from build123d import *

# Parameters (mm, degrees)
SKETCH1_R           = 4
BOSS_EXTRUDE1_DEPTH = 50
SKETCH2_R           = 1.5
CUT_EXTRUDE1_DEPTH  = 5
FILLET1_R           = 2
SKETCH3_R           = 1.5
CUT_EXTRUDE2_DEPTH  = 4


with BuildPart() as part:
    # Sketch1 → Boss-Extrude1 (new, symmetric)
    with BuildSketch(Plane.XY):
        Circle(SKETCH1_R)
    extrude(amount=BOSS_EXTRUDE1_DEPTH, both=True)

    # Sketch2 → Cut-Extrude1 (cut)
    with BuildSketch(Plane(origin=(0, 0, 0), x_dir=(0, 0, -1), z_dir=(1, 0, 0))):
        with Locations((-45, 0)):
            Circle(SKETCH2_R)
        with Locations((45, 0)):
            Circle(SKETCH2_R)
    extrude(amount=CUT_EXTRUDE1_DEPTH, mode=Mode.SUBTRACT)

    # Fillet1
    fillet1_edges = [part.edges().sort_by_distance(p)[0] for p in [
        (-4, 0, -50),
        (-4, 0, 50),
    ]]
    fillet(fillet1_edges, radius=FILLET1_R)

    # Sketch3 → Cut-Extrude2 (cut)
    with BuildSketch(Plane(origin=(0, 0, 0), x_dir=(1, 0, 0), z_dir=(0, 1, 0))):
        with Locations(Location((0, 45, 0), (0, 0, 90))):
            Circle(SKETCH3_R)
        with Locations(Location((0, -45, 0), (0, 0, 90))):
            Circle(SKETCH3_R)
    extrude(amount=CUT_EXTRUDE2_DEPTH, mode=Mode.SUBTRACT)


solid = part.part
Design review of the part built by this model. Coordinates are the model's own, in mm. A direction names the side the tool comes from. Give positions to 0.01 mm unless a question says otherwise; leave off trailing zeros. Write each loop counter-clockwise with the first axis right and the second up, starting at its lowest first coordinate (ties: lowest second). Pieces come first, ordered by that corner, then holes. Notation, with made-up numbers: M 69.25,-39 L 116.25,-39 A21 cw 116.25,-14 Z; hole C 43,-39.75 d5. An arc over 180 degrees is marked long. Return JSON: item names as keys, results as strings. Group by question number.
Item 1: Take a section at B-B (z = -35.5). Give the boundary of the cut face in (x, y), plus the area to 3 significant figures.
Item 2: Clearance check with flat-ended pins moving along their axes: pin 1 Ø1.7 at (y, z) = (-1, 45.5) entering from +X; pin 2 Ø2 at (x, z) = (1.5, 30) entering from -Y; pin 3 Ø0.8 at (x, z) = (-1, 45) entering from +Y. State where each tip first meets the part, or that it passes through.
Item 3: Wall thickness on line 1 along Z through (x, y) = (1.4, 0); line 2 along Z through (x, y) = (-0.75, 2); line 3 along X through (y, z) = (-0.25, -45.5): over which ranges is each line inside the solid? List them lowest first.
Item 4: The part is to be moulded in two halves that separate along X. For faces 3 (the cylindrical face through (-0.867, -3.905, 0.672)), 4 (the cylindrical face through (-1.487, 1.972, 45.195)), 5 (the cylindrical face through (-1.487, 1.972, -44.805)), 6 (the cylindrical face through (1.972, -1.464, 45.325)), say which applies: pulls with the +X half, pulls with the -X half, needs draft (parallel to the pull), parting line crosses it, or undercut.
Item 5: Tool access review of faces 1 (the flat face through (0, 0, 50)), 2 (the cylindrical face through (1.972, -1.464, -44.675)): name each direction out of +Z, -Z, +X, -X, +Y, -Y from which nothing blocks a thin tool from reaching the whole face with its end or side.
Item 6: Take a section at A-A (z = 45). Give the boundary of the cut face in (x, y).
Return value:
{
 "1": {"outline": "C 0,0 d8", "area": "50.3 mm2"},
 "2": {"pin 1": "stops at x = 3.93", "pin 2": "stops at y = -3.97", "pin 3": "stops at y = 0"},
 "3": {"line 1": "z = -50 to -46.5, -43.5 to 43.5, 46.5 to 50", "line 2": "z = -50 to -46.3, -43.7 to 43.7, 46.3 to 50", "line 3": "x = -3.99 to 0"},
 "4": {"face 3": "parting line crosses it", "face 4": "undercut", "face 5": "undercut", "face 6": "needs draft"},
 "5": {"face 1": "+Z, +X, -X, +Y, -Y", "face 2": "+X"},
 "6": {"outline": "M -1.5,0 L -1.5,3.71 A4 ccw long 3.71,-1.5 L 0,-1.5 L 0,0 Z; M 1.5,1.5 L 3.71,1.5 A4 ccw 1.5,3.71 Z"}
}
